Read the model definition and answer for the solid it produces. Units are mm, in the model's axes. Face numbers are marked on the shaded views. Coordinates: 2 decimals unless noted, no trailing zeros. Loops run counter-clockwise (first coordinate to the right, second up) from the corner with the lowest first, then second, coordinate; pieces in that order, holes last.
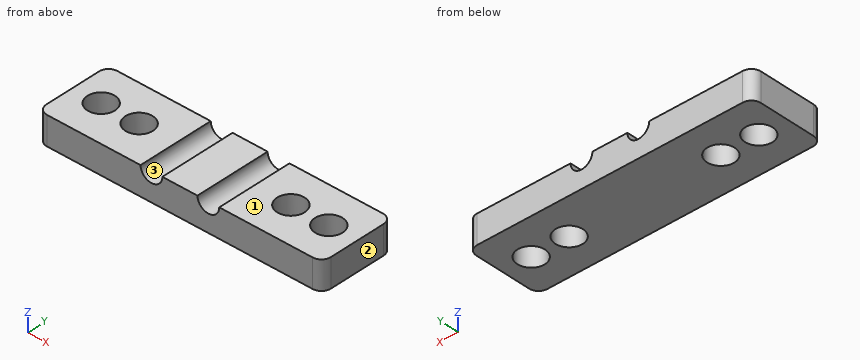
from build123d import *

# Parameters (mm, degrees)
F0_W     = 6
F0_H     = 8
F0_W_2   = 18
F1_DEPTH = 3
F2_D     = 2.9
F4_D     = 2.3
F5_R     = 1


with BuildPart() as f1:
    # F0 (on Top) → F1 (new body)
    with BuildSketch(Plane.XY):
        Rectangle(F0_W, F0_H)
        with Locations((12, 0)):
            Rectangle(F0_W_2, F0_H)
        with Locations((24, 0)):
            Rectangle(F0_W, F0_H)
    extrude(amount=-F1_DEPTH)

    # F2 (through all)
    with Locations(Plane.XY):
        with Locations((0, 0), (4, 0), (20, 0), (24, 0)):
            Hole(F2_D / 2)

    # F4 (through all)
    with Locations(Plane.XZ.offset(4)):
        with Locations((9, 0), (15, 0)):
            Hole(F4_D / 2)

    # F5
    f5_edges = [f1.edges().sort_by_distance(p)[0] for p in [
        (-3, -4, -1.5),
        (27, -4, -1.5),
        (27, 4, -1.5),
        (-3, 4, -1.5),
    ]]
    fillet(f5_edges, radius=F5_R)


solid = f1.part
Q1. A flat-ended cylindrical pin translates along its axis: pin 1 Ø4.5 at (x, y) = (4, 0) entering from -Z. Find the tip coordinate at first contact, or state that the pin passes through.
Findings below:
pin 1: stops at z = -3
Q2. A cutting plane is placed at B-B (y = -1.75). Give the vertices of the cut face in (x, z).
Findings below:
outline: (-3, -3) - (27, -3) - (27, 0) - (16.15, 0) arc R1.15 cw to (13.85, 0) - (10.15, 0) arc R1.15 cw to (7.85, 0) - (-3, 0) - close
Q3. A cutting plane is placed at A-A (x = 24). Give the vertices of the cut face in (y, z).
Findings below:
outline: (-4, -3) - (-1.45, -3) - (-1.45, 0) - (-4, 0) - close; (1.45, -3) - (4, -3) - (4, 0) - (1.45, 0) - close
Q4. A cutting plane is placed at D-D (y = 0). Give the vertices of the cut face in (x, z), then the cut area to 3 significant figures.
Findings below:
outline: (-3, -3) - (-1.45, -3) - (-1.45, 0) - (-3, 0) - close; (1.45, -3) - (2.55, -3) - (2.55, 0) - (1.45, 0) - close; (5.45, -3) - (18.55, -3) - (18.55, 0) - (16.15, 0) arc R1.15 cw to (13.85, 0) - (10.15, 0) arc R1.15 cw to (7.85, 0) - (5.45, 0) - close; (21.45, -3) - (22.55, -3) - (22.55, 0) - (21.45, 0) - close; (25.45, -3) - (27, -3) - (27, 0) - (25.45, 0) - close
area: 51.0 mm2
Q5. A cutting plane is placed at C-C (z = -2.05). Give the vertices of the cut face in (x, y), then the cut area to 3 significant figures.
Findings below:
outline: (-3, -3) arc R1 ccw to (-2, -4) - (26, -4) arc R1 ccw to (27, -3) - (27, 3) arc R1 ccw to (26, 4) - (-2, 4) arc R1 ccw to (-3, 3) - close; hole circle Ø2.9 at (0, 0); hole circle Ø2.9 at (4, 0); hole circle Ø2.9 at (20, 0); hole circle Ø2.9 at (24, 0)
area: 213 mm2
Q6. Straight lines are drawn through the part: probe 1 along Y at (x, z) = (4, -1.2); probe 2 along X at (y, z) = (-3.25, -0.35); probe 3 along X at (y, z) = (0.25, -1.9). For each, find the intervals that lie inside material, in ascending order.
Findings below:
probe 1: y = -4 to -1.45, 1.45 to 4
probe 2: x = -2.97 to 7.9, 10.1 to 13.9, 16.1 to 26.97
probe 3: x = -3 to -1.43, 1.43 to 2.57, 5.43 to 18.57, 21.43 to 22.57, 25.43 to 27
Q7. Determine the mould class of the marked faces 1, 2 and 3 for opening direction X: +X half, -X half, draft (parallel to the pull), parting line (faces both ways), or undercut.
Findings below:
face 1: draft
face 2: +X half
face 3: undercut
